```python
from build123d import *

# Parameters (mm, degrees)
F0_R     = 6
F0_R_2   = 5.5
F0_R_3   = 3
F1_DEPTH = 25
F0_R_4   = 6.5
F2_DEPTH = 2
F0_R_5   = 1.5
F3_DEPTH = 2.4
F4_R     = 6.25
F5_DEPTH = 75
F6_DEPTH = 40


# Not quite as in the source:
# - a fillet or chamfer that OpenCascade refuses, or shapes differently, is made with other operations: its cross-section is extruded or revolved along the edge and cut away or added


with BuildPart() as f1:
    # F0 (on Top) → F1 (new body)
    with BuildSketch(Plane.XY):
        with Locations((-55, 0)):
            Circle(F0_R)
        with Locations((-55, 0)):
            Circle(F0_R_2, mode=Mode.SUBTRACT)
        with Locations((-55, 0)):
            Circle(F0_R_2)
        with Locations((-55, 0)):
            Circle(F0_R_3, mode=Mode.SUBTRACT)
    extrude(amount=F1_DEPTH)

    # F0 (on Top) → F2 (join)
    with BuildSketch(Plane.XY):
        with Locations((-55, 0)):
            Circle(F0_R_4)
        with Locations((-55, 0)):
            Circle(F0_R, mode=Mode.SUBTRACT)
    extrude(amount=F2_DEPTH)

    # F0 (on Top) → F3 (join)
    with BuildSketch(Plane.XY):
        with Locations((-55, 0)):
            Circle(F0_R_2)
        with Locations((-55, 0)):
            Circle(F0_R_3, mode=Mode.SUBTRACT)
        with Locations((-55, 0)):
            Circle(F0_R_3)
        with Locations((-55, 0)):
            Circle(F0_R_5, mode=Mode.SUBTRACT)
    extrude(amount=-F3_DEPTH)

    # F4 (on Right) → F5 (join)
    with BuildSketch(Plane.YZ):
        with Locations((0, 25.1302048564)):
            Circle(F4_R)
    extrude(amount=-F5_DEPTH)

    # F0 (on Top) → F6 (cut)
    with BuildSketch(Plane.XY):
        with Locations((-55, 0)):
            Circle(F0_R_3)
        with Locations((-55, 0)):
            Circle(F0_R_5, mode=Mode.SUBTRACT)
        with Locations((-55, 0)):
            Circle(F0_R_5)
    extrude(amount=F6_DEPTH, mode=Mode.SUBTRACT)

    # F7: fillet of radius 1 on 1 edges, made by hand

    # F7_s1 → F7_t2 (revolve, cut)
    with BuildSketch(Plane.XZ):
        with BuildLine():
            ThreePointArc((-49, 2), (-48.6339745962, 1.6339745962), (-48.5, 1.1339745962))
            Line((-48.5, 1.1339745962), (-48.5, 2))
            Line((-48.5, 2), (-49, 2))
        make_face()
    revolve(axis=Axis((-55, 0, 2), (0, 0, 1)), mode=Mode.SUBTRACT)

    # F8: F1 across plane


with BuildPart() as f1_1:
    add(f1.part)
    add(f1.part.mirror(Plane.YZ))


solid = f1_1.part
```
CAD build for the part. Positions are in the model's coordinates, mm. A direction names the side the tool comes from. Round coordinates to 2 decimals unless told otherwise and drop trailing zeros. Order: outer loops, then holes, each group sorted by start corner. A loop starts at its lowest first (then second) coordinate and runs counter-clockwise, first axis right, second up. Notation, with made-up numbers: (-23.75, -35.75) - (2.25, -35.75) arc R31 ccw to (2.25, -0.75) - close; hole circle Ø6 at (9, 68). An arc over 180 degrees is marked (long way). Answer in a Markdown table with one row per item. Add a question column.
(1) Probe L1, parallel to X at y = -0.25, z = 17; L2, parallel to X at y = -1, z = 3.5; L3, parallel to Y at x = 55, z = -0.7. List the from-to ranges inside material, lowest first. Write a range as [from, to].
(2) Drop flat-ended pins along their axis: pin 1 Ø5.5 at (x, y) = (-55, 0) entering from +Z; pin 2 Ø3 at (x, z) = (3.5, 23) entering from -Y; pin 3 Ø1.8 at (x, y) = (55, 0) entering from +Z; pin 4 Ø1 at (x, z) = (-33, 23) entering from -Y. Give the stop position or say it passes through.
(3) Band-saw the part on B-B on z = 6. List the corners of the cut face in (x, y), and give its area (3 significant figures).
(4) Band-saw the part on C-C on y = 0. Count the separate pieces of the cut face and the enclosed holes in it, and give its area (3 significant figures).
(5) Mould opens along Y. For faces 5 (the face through (53.57, 0.45, -1.18)), 6 (the face through (-48.8, 1.95, 0.56)), 7 (the face through (53.9, 1.3, -2.4)) say: +Y half, -Y half, draft (parallel to the pull), parting line (faces both ways), or undercut.
(6) 3-axis set-ups, long thin cutter, end or side, ignore diameter. For faces 1 (the face through (-53.7, -1.3, 0)), 2 (the face through (-60, 3, 0)), 3 (the face through (-1.05, -0.814, 31.327)), 4 (the face through (-53.57, 0.45, -1.18)): which of +Z, -Z, +X, -X, +Y, -Y reach the whole face in a straight line?
(7) Band-saw the part on A-A on x = 55. List the corners of the cut face in (y, z), and give its area (3 significant figures).
Data:
| question | item | result |
|---|---|---|
| 1 | L1 | x = [-60.99, -57.99], [-52.01, -49.01], [49.01, 52.01], [57.99, 60.99] |
| 1 | L2 | x = [-60.92, -57.83], [-52.17, -49.08], [49.08, 52.17], [57.83, 60.92] |
| 1 | L3 | y = [-5.5, -1.5], [1.5, 5.5] |
| 2 | pin 1 | stops at z = 0 |
| 2 | pin 2 | stops at y = -6.22 |
| 2 | pin 3 | passes through |
| 2 | pin 4 | stops at y = -6.03 |
| 3 | outline | circle Ø12 at (-55, 0); circle Ø12 at (55, 0); hole circle Ø6 at (-55, 0); hole circle Ø6 at (55, 0) |
| 3 | area | 170 mm^2 |
| 4 | separate pieces | 3 |
| 4 | enclosed holes | 0 |
| 4 | area | 1,990 mm^2 |
| 5 | face 5 | undercut |
| 5 | face 6 | parting line |
| 5 | face 7 | draft |
| 6 | face 1 | +Z |
| 6 | face 2 | -Z |
| 6 | face 3 | none |
| 6 | face 4 | +Z, -Z |
| 7 | outline | (-6.5, 0) - (-5.5, 0) - (-5.5, -2.4) - (-1.5, -2.4) - (-1.5, 0) - (-3, 0) - (-3, 30.61) arc R6.25 ccw to (-6, 23.38) - (-6, 2) arc R1 ccw to (-6.5, 1.13) - close; (1.5, -2.4) - (5.5, -2.4) - (5.5, 0) - (6.5, 0) - (6.5, 1.13) arc R1 ccw to (6, 2) - (6, 23.38) arc R6.25 ccw to (3, 30.61) - (3, 0) - (1.5, 0) - close |
| 7 | area | 198 mm^2 |
